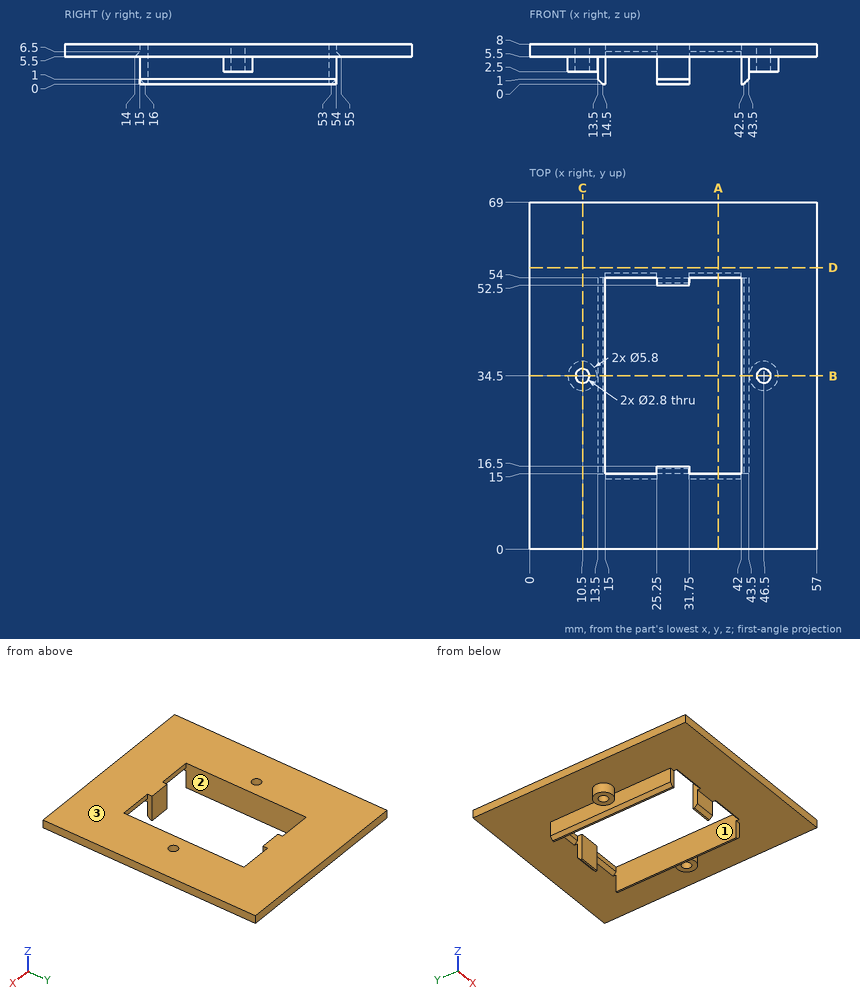
Here's the drawing with two shaded views (mm, measured from the low corner). I have some questions. Round coordinates to 2 decimals unless told otherwise and drop trailing zeros. Order: outer loops, then holes, each group sorted by start corner. A loop starts at its lowest first (then second) coordinate and runs counter-clockwise, first axis right, second up. Notation, with made-up numbers: M 81.5,16 L 100.5,16 A18 cw 100.5,44 Z; hole C 84.25,52 d8. An arc over 180 degrees is marked long. Use CSV: the item, a comma, the result in double quotes.
1) I'm going to push flat-ended pins straight in: P1, Ø0.8, axis at y = 54, z = 3, coming from the -X side; P2, Ø1.3, axis at x = 28.5, z = 4, coming from the -Y side; P3, Ø3.5, axis at y = 27.5, z = 2.5, coming from the +X side. Where does each tip first touch, or does it pass through?
Taken from the geometry:
P1,"x = 13.5"
P2,"y = 15"
P3,"x = 43.5"
2) I want a section at C-C (x = 10.5). List the corners of the cut face in (y, z) for me, then the cut area to 4 significant figures.
Taken from the geometry:
outline,"M 0,5.5 L 31.6,5.5 L 31.6,2.5 L 33.1,2.5 L 33.1,8 L 0,8 Z; M 35.9,2.5 L 37.4,2.5 L 37.4,5.5 L 69,5.5 L 69,8 L 35.9,8 Z"
area,"174.5 mm^2"
3) I want a section at D-D (y = 56). List the corners of the cut face in (x, z) for me, then the cut area to 4 significant figures.
Taken from the geometry:
outline,"M 0,5.5 L 57,5.5 L 57,8 L 0,8 Z"
area,"142.5 mm^2"
4) If we mould it in two halves opening along X, with no side actions, what happens to the marked faces 1, 2 and 3? For each: pulls with the +X half, pulls with the -X half, needs draft (parallel to the pull), parting line crosses it, or undercut.
Taken from the geometry:
face 1,"undercut"
face 2,"undercut"
face 3,"needs draft"
5) I want a section at B-B (y = 34.5). Count the separate pieces of the cut face and the enclosed holes in it, then the cut area to 3 significant figures.
Taken from the geometry:
separate pieces,"4"
enclosed holes,"0"
area,"94.5 mm^2"
6) I need wall thicknesses on line 1 along X through (y, z) = (34, 1); line 2 along X through (y, z) = (50, 6.5); line 3 along Y through (x, z) = (10.5, 4.05). Which ranges of each line are inside material? Lowest first, please. Write a range as [from, to].
Taken from the geometry:
line 1,"[13.5, 15], [42, 43.5]"
line 2,"[0, 15], [42, 57]"
line 3,"[31.6, 33.1], [35.9, 37.4]"
7) I want a section at A-A (x = 37.5). List the corners of the cut face in (y, z) for me.
Taken from the geometry:
outline,"M 0,5.5 L 14,5.5 L 15,6.5 L 15,8 L 0,8 Z; M 54,6.5 L 55,5.5 L 69,5.5 L 69,8 L 54,8 Z"
